from build123d import *

# Parameters (mm, degrees)
SCALE1_SCALE = 0.266666667


with BuildPart() as part:
    # Sketch1 → Revolve1 (revolve)
    with BuildSketch(Plane(origin=(0, 0, 0), x_dir=(0, 0, -1), z_dir=(1, 0, 0))):
        with BuildLine():
            Line((25, -8), (25, -4.538997687))
            ThreePointArc((25, -4.538997687), (25.088639197, -4.127389271), (25.338842975, -3.788750135))
            ThreePointArc((25.338842975, -3.788750135), (27.05, 0), (25.338842975, 3.788750135))
            ThreePointArc((25.338842975, 3.788750135), (25.088639197, 4.127389271), (25, 4.538997687))
            Line((25, 4.538997687), (25, 8))
            ThreePointArc((25, 8), (25.292893219, 8.707106781), (26, 9))
            Line((26, 9), (30, 9))
            Line((30, 9), (30, -9))
            Line((30, -9), (26, -9))
            ThreePointArc((26, -9), (25.292893219, -8.707106781), (25, -8))
        make_face()
    revolve(axis=Axis((0, 0, 0), (0, 1, 0)))


with BuildPart() as part_1:
    # Scale1: scaled about (0, 0, 0)
    add(part.part.scale(SCALE1_SCALE))


solid = part_1.part
Geometry: final body of the model. Coordinates: model frame, mm. Round coordinates to 2 decimals unless told otherwise and drop trailing zeros. Loops run counter-clockwise (first coordinate to the right, second up) from the corner with the lowest first, then second, coordinate; pieces in that order, holes last.
Q1. Section B-B on z = 0. Return loops of the section in (x, y).
Q2. Section A-A on x = 0. Return loops of the section in (y, z), plus the area to 3 significant figures.
Q3. Pin query (flat end, axial travel): P1, Ø2, axis at y = 1, z = 5.5, coming from the +X side; P2, Ø1.5, axis at x = -3, y = 0, coming from the -Z side; P3, Ø1, axis at y = 0.5, z = 2.5, coming from the +X side. Return the tip coordinate at first contact, or that it passes through.
Q4. Material intervals for L1, parallel to Z at x = 0, y = -1.5; L2, parallel to X at y = -0.75, z = -3.5, sorted ascending.
Q5. Pull-direction query (X, two-part tool) for faces 1 (the cylindrical face through (4.06, -1.67, 5.29)), 2 (the flat face through (-7, 2.4, -2)), 3 (the cylindrical face through (7.81, -0.03, 1.73)); classes: released by +X, released by -X, zero draft, split by the parting line, or undercut.
Evaluation:
1. outline: (-8, -2.4) - (-6.93, -2.4) arc R0.27 ccw to (-6.67, -2.13) - (-6.67, -1.21) arc R0.27 ccw to (-6.76, -1.01) arc R1.35 cw to (-6.76, 1.01) arc R0.27 ccw to (-6.67, 1.21) - (-6.67, 2.13) arc R0.27 ccw to (-6.93, 2.4) - (-8, 2.4) - close; (6.67, -2.13) arc R0.27 ccw to (6.93, -2.4) - (8, -2.4) - (8, 2.4) - (6.93, 2.4) arc R0.27 ccw to (6.67, 2.13) - (6.67, 1.21) arc R0.27 ccw to (6.76, 1.01) arc R1.35 cw to (6.76, -1.01) arc R0.27 ccw to (6.67, -1.21) - close
2. outline: (-2.4, -8) - (2.4, -8) - (2.4, -6.93) arc R0.27 ccw to (2.13, -6.67) - (1.21, -6.67) arc R0.27 ccw to (1.01, -6.76) arc R1.35 cw to (-1.01, -6.76) arc R0.27 ccw to (-1.21, -6.67) - (-2.13, -6.67) arc R0.27 ccw to (-2.4, -6.93) - close; (-2.4, 6.93) arc R0.27 ccw to (-2.13, 6.67) - (-1.21, 6.67) arc R0.27 ccw to (-1.01, 6.76) arc R1.35 cw to (1.01, 6.76) arc R0.27 ccw to (1.21, 6.67) - (2.13, 6.67) arc R0.27 ccw to (2.4, 6.93) - (2.4, 8) - (-2.4, 8) - close
2. area: 11.1 mm2
3. P1: stops at x = 6.61
3. P2: stops at z = -7.68
3. P3: stops at x = 7.75
4. L1: z = -8 to -6.67, 6.67 to 8
4. L2: x = -7.19 to -6.05, 6.05 to 7.19
5. face 1: undercut
5. face 2: zero draft
5. face 3: split by the parting line
